Geometry: final body of the model. Coordinates: model frame, mm. A direction names the side the tool comes from. Give positions to 0.01 mm unless a question says otherwise; leave off trailing zeros. Loops run counter-clockwise (first coordinate to the right, second up) from the corner with the lowest first, then second, coordinate; pieces in that order, holes last.
from build123d import *

# Parameters (mm, degrees)
F_4_40_TAPPED_HOLE1_D     = 2.2606
F_4_40_TAPPED_HOLE1_DEPTH = 6.35
F_4_40_TAPPED_HOLE1_TIP   = 0.679152758
FILLET1_R                 = 0.79375
CHAMFER1_SIZE             = 0.762
CHAMFER2_SIZE             = 0.508


with BuildPart() as part:
    # Sketch1 → Revolve1 (revolve)
    with BuildSketch(Plane(origin=(0, 0, 0), x_dir=(1, 0, 0), z_dir=(0, 1, 0))):
        with BuildLine():
            Line((0, 0), (0, 9.525))
            ThreePointArc((0, 9.525), (6.735192091, 6.735192091), (9.525, 0))
            Line((9.525, 0), (0, 0))
        make_face()
    revolve(axis=Axis((0, 0, 0), (0, 0, -1)))

    # #4-40 Tapped Hole1
    with Locations(Plane.XY):
        with Locations((0, 0)):
            Hole(F_4_40_TAPPED_HOLE1_D / 2, depth=F_4_40_TAPPED_HOLE1_DEPTH)
            with Locations((0, 0, -(F_4_40_TAPPED_HOLE1_DEPTH + F_4_40_TAPPED_HOLE1_TIP / 2))):  # 118° drill point
                Cone(0, F_4_40_TAPPED_HOLE1_D / 2, F_4_40_TAPPED_HOLE1_TIP, mode=Mode.SUBTRACT)

    # Fillet1
    fillet1_edges = [part.edges().sort_by_distance(p)[0] for p in [
        (0, 1.1303, -6.35),
    ]]
    fillet(fillet1_edges, radius=FILLET1_R)

    # Chamfer1
    # the kernel refuses this chamfer: 0.762 mm, written as the material it takes off along each edge
    with BuildSketch(Plane(origin=(0, 0, 0), x_dir=(1, 0, 0), z_dir=(0, 1, 0))) as chamfer1_piece_1:
        with BuildLine():
            Line((9.525 - CHAMFER1_SIZE, 0), (9.496699923, 0.733699923))
            ThreePointArc((9.496699923, 0.733699923), (9.517517871, 0.37746333), (9.525, 0))
            Line((9.525, 0), (9.525 - CHAMFER1_SIZE, 0))
        make_face()
    revolve(axis=Axis((0, 0, 0), (0, 0, -1)), mode=Mode.SUBTRACT)

    # Chamfer2
    chamfer2_edges = [part.edges().sort_by_distance(p)[0] for p in [
        (1.1303, 0, 0),
    ]]
    chamfer(chamfer2_edges, length=CHAMFER2_SIZE)


solid = part.part
Item 1: Ray query, probe 1 along Y at (x, z) = (0, -3.45); probe 2 along Y at (x, z) = (0, -4.5); probe 3 along Y at (x, z) = (1.5, -8.5). Return the intervals inside material, ascending.
Values follow:
probe 1: y = -8.88 to -1.13, 1.13 to 8.88
probe 2: y = -8.39 to -1.13, 1.13 to 8.39
probe 3: y = -4.03 to 4.03
Item 2: Section query A-A on z = -3.75. Return loops of the section in (x, y), plus the area to 3 significant figures.
Values follow:
outline: circle Ø17.51 at (0, 0); hole circle Ø2.26 at (0, 0)
area: 237 mm2
Item 3: Section query B-B on z = -8.25. Return loops of the section in (x, y).
Values follow:
outline: circle Ø9.52 at (0, 0)
Item 4: Set-up query: faces 1 (the face through (2, 0, 0)), 2 (the face through (0.245, -1.103, -3.243)). Return all of +Z, -Z, +X, -X, +Y, -Y with unobstructed straight access to the full face (end or side cutting, diameter ignored); none if empty.
Values follow:
face 1: +Z, +X, -X, +Y, -Y
face 2: +Z
Item 5: Section query C-C on z = -5.5. Return loops of the section in (x, y), plus the area to 3 significant figures.
Values follow:
outline: circle Ø15.55 at (0, 0); hole circle Ø2.26 at (0, 0)
area: 186 mm2
Item 6: Pin query (flat end, axial travel): pin 1 (1.5 mm diameter, centred on y = 5.5, z = -1.5, fed in from -X); pin 2 (1.5 mm diameter, centred on y = -6, z = -5, fed in from +X); pin 3 (1.5 mm diameter, centred on y = -3.5, z = -6.5, fed in from -X). Return the tip coordinate at first contact, or that it passes through.
Values follow:
pin 1: stops at x = -8.14
pin 2: stops at x = 6.39
pin 3: stops at x = -6.84
